Design review of the part shown in the three views and the two pictorial views. Dimensions are in mm from the part's minimum x, y and z. A direction names the side the tool comes from. Round coordinates to 2 decimals unless told otherwise and drop trailing zeros. Loops run counter-clockwise (first coordinate to the right, second up) from the corner with the lowest first, then second, coordinate; pieces in that order, holes last. Notation, with made-up numbers: M 55,63 L 106,63 A16 ccw 106,89 Z; hole C 2.5,9.25 d7. An arc over 180 degrees is marked long. Answer as CSV lines item,"result". Start each with the question number.
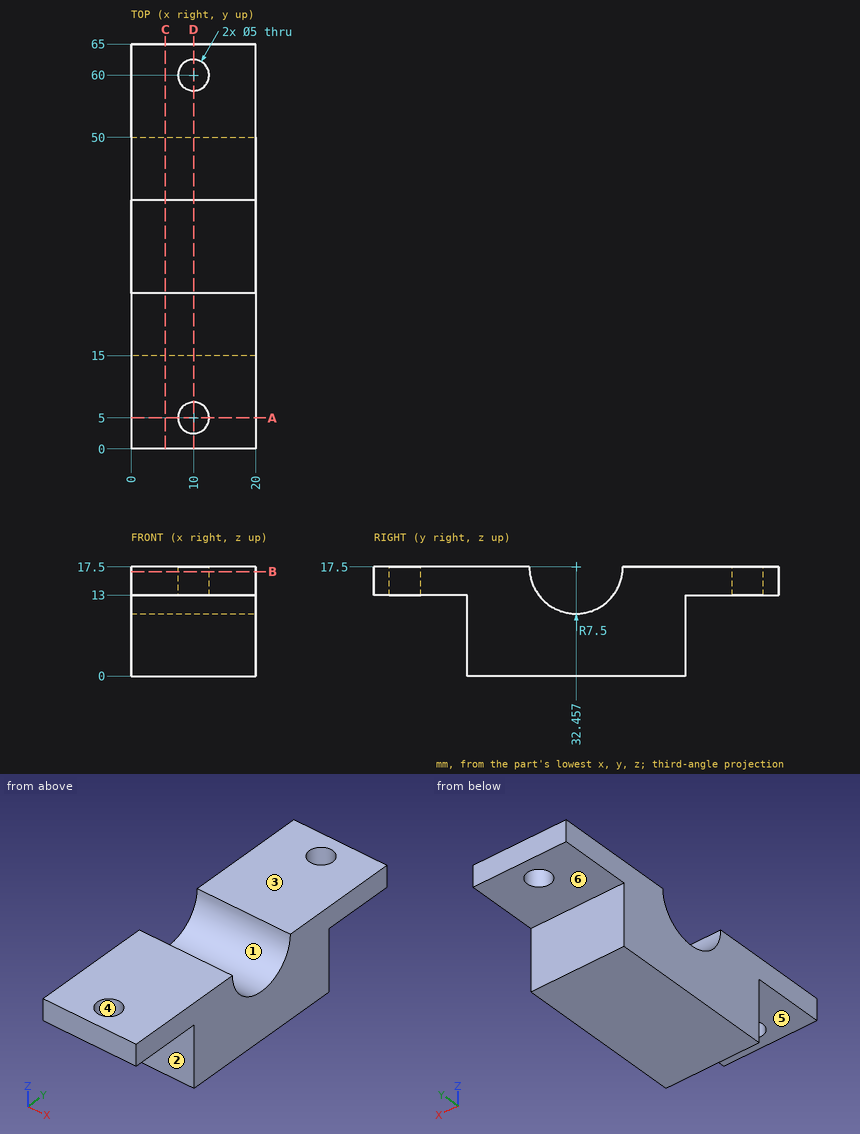
Item 1: Consider section C-C, the plane x = 5.5. Write out the cut boundary in (y, z), then the cut area to 3 significant figures.
Item 2: Consider section D-D, the plane x = 10. Write out the cut boundary in (y, z), then the cut area to 3 significant figures.
Item 3: Consider section B-B, the plane z = 16.75. Write out the cut boundary in (x, y).
Item 4: Tool access review of the marked faces 4, 5 and 6: name each direction out of +Z, -Z, +X, -X, +Y, -Y from which nothing blocks a thin tool from reaching the whole face with its end or side.
Item 5: To check wall thickness, follow line 1 (X direction, y = 60, z = 15.6); line 2 (Y direction, x = 10, z = 15.35); line 3 (Y direction, x = 10, z = 14.9). State the ranges of each line that lie inside material, in increasing order.
Item 6: The part is to be moulded in two halves that separate along Y. For the marked faces 1, 2 and 3, say which applies: +Y half, -Y half, draft (parallel to the pull), parting line (faces both ways), or undercut.
Item 7: Insertion check: pin 1 Ø3 at (x, y) = (10, 60) entering from +Z; pin 2 Ø4 at (x, z) = (11.5, 4) entering from +Y; pin 3 Ø7.5 at (x, y) = (6.5, 6.5) entering from -Z; pin 4 Ø10.5 at (x, z) = (13.5, 5) entering from -Y. Each pin has a flat end and moves straight along its axis. Give the tip position at first contact, or say it passes through.
Item 8: Consider section A-A, the plane y = 5. Write out the cut boundary in (x, z).
Found:
1,outline,"M 0,13 L 15,13 L 15,0 L 50,0 L 50,13 L 65,13 L 65,17.5 L 39.96,17.5 A7.5 cw 24.96,17.5 L 0,17.5 Z"
1,area,"659 mm^2"
2,outline,"M 0,13 L 2.5,13 L 2.5,17.5 L 0,17.5 Z; M 7.5,13 L 15,13 L 15,0 L 50,0 L 50,13 L 57.5,13 L 57.5,17.5 L 39.96,17.5 A7.5 cw 24.96,17.5 L 7.5,17.5 Z; M 62.5,13 L 65,13 L 65,17.5 L 62.5,17.5 Z"
2,area,"614 mm^2"
3,outline,"M 0,0 L 20,0 L 20,24.99 L 0,24.99 Z; M 0,39.92 L 20,39.92 L 20,65 L 0,65 Z; hole C 10,5 d5; hole C 10,60 d5"
4,face 4,"+Z, -Z"
4,face 5,"-Z, +X, -X, -Y"
4,face 6,"-Z, +X, -X, +Y"
5,line 1,"x = 0 to 7.5, 12.5 to 20"
5,line 2,"y = 0 to 2.5, 7.5 to 25.27, 39.64 to 57.5, 62.5 to 65"
5,line 3,"y = 0 to 2.5, 7.5 to 25.42, 39.49 to 57.5, 62.5 to 65"
6,face 1,"undercut"
6,face 2,"-Y half"
6,face 3,"draft"
7,pin 1,"passes through"
7,pin 2,"stops at y = 50"
7,pin 3,"stops at z = 13"
7,pin 4,"stops at y = 15"
8,outline,"M 0,13 L 7.5,13 L 7.5,17.5 L 0,17.5 Z; M 12.5,13 L 20,13 L 20,17.5 L 12.5,17.5 Z"
